from build123d import *

# Parameters (mm, degrees)
F0_W     = 203.2
F0_H     = 101.6
F1_DEPTH = 101.6
F2_W     = 101.6
F2_H     = 76.2
F3_DEPTH = 50.8
F5_DEPTH = 50.8
F7_DEPTH = 50.8


with BuildPart() as f1:
    # F0 (on Front) → F1 (new body)
    with BuildSketch(Plane.XZ):
        with Locations((-39.505829, 21.651511)):
            Rectangle(F0_W, F0_H)
    extrude(amount=F1_DEPTH)

    # F2 (on face) → F3 (cut)
    with BuildSketch(Plane.XZ.offset(101.6)):
        with Locations((-39.505829, 34.351511)):
            Rectangle(F2_W, F2_H)
    extrude(amount=-F3_DEPTH, mode=Mode.SUBTRACT)

    # F4 (on face) → F5 (cut)
    with BuildSketch(Plane.YZ.offset(-90.305829)):
        Polygon((-101.6, 72.451511), (-101.6, -3.748489), (-50.8, 72.451511), align=None)
    extrude(amount=-F5_DEPTH, mode=Mode.SUBTRACT)

    # F6 (on face) → F7 (cut)
    with BuildSketch(Plane(origin=(11.294171, 0, 0), x_dir=(0, -1, 0), z_dir=(-1, 0, 0))):
        Polygon((101.6, 72.451511), (50.8, 72.451511), (101.6, -3.748489), align=None)
    extrude(amount=-F7_DEPTH, mode=Mode.SUBTRACT)


solid = f1.part
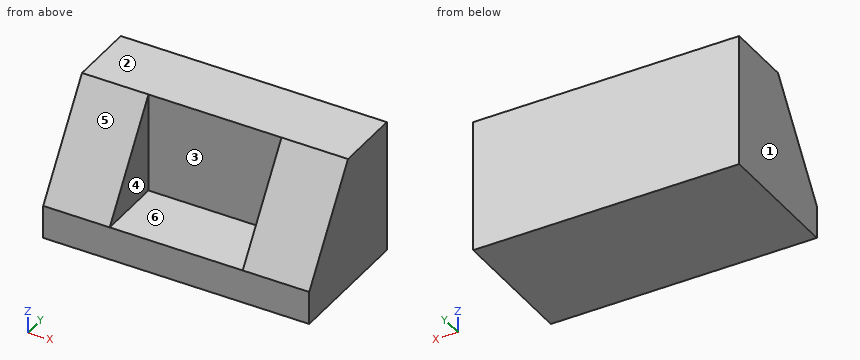
Input: part model. Units: mm. Frame: model coordinates. Face numbers are marked on the shaded views. A direction names the side the tool comes from. Give positions to 0.01 mm unless a question says otherwise; leave off trailing zeros. Loops run counter-clockwise (first coordinate to the right, second up) from the corner with the lowest first, then second, coordinate; pieces in that order, holes last. Notation, with made-up numbers: M 78.25,-2.5 L 114.25,-2.5 A29 cw 114.25,36.5 Z; hole C 45,62.5 d4. An arc over 180 degrees is marked long. Use one line per item in the form item = value.
1. Section query D-D, the plane x = -65. Return the cut outline in (y, z), and give its area (3 significant figures).
Numbers:
outline = M -101.6,-29.15 L 0,-29.15 L 0,72.45 L -50.8,72.45 L -50.8,-3.75 L -101.6,-3.75 Z
area = 6,450 mm²
2. Line query: L1, parallel to X at y = -59, z = 11; L2, parallel to Y at x = -23, z = -3; L3, parallel to Z at x = -5, y = -56. Output: solid intervals per line, ascending.
Numbers:
L1 = -141.11 to -90.31, 11.29 to 62.09
L2 = -50.8 to 0
L3 = -29.15 to -3.75
3. Section query A-A, the plane x = -100.5. Return the cut outline in (y, z), and give its area (3 significant figures).
Numbers:
outline = M -101.6,-29.15 L 0,-29.15 L 0,72.45 L -50.8,72.45 L -101.6,-3.75 Z
area = 8,390 mm²
4. Section query B-B, the plane z = 58.5. Return the cut outline in (x, y).
Numbers:
outline = M -141.11,-60.1 L -90.31,-60.1 L -90.31,-50.8 L 11.29,-50.8 L 11.29,-60.1 L 62.09,-60.1 L 62.09,0 L -141.11,0 Z
5. Section query C-C, the plane y = -65.5. Return the cut outline in (x, z).
Numbers:
outline = M -141.11,-29.15 L 62.09,-29.15 L 62.09,50.4 L 11.29,50.4 L 11.29,-3.75 L -90.31,-3.75 L -90.31,50.4 L -141.11,50.4 Z
6. Pull-direction query (X, two-part tool) for the marked faces 1, 2, 3 and 4; classes: released by +X, released by -X, zero draft, split by the parting line, or undercut.
Numbers:
face_1 = released by -X
face_2 = zero draft
face_3 = undercut
face_4 = undercut
7. Reachability of the marked faces 5 and 6 from +Z, -Z, +X, -X, +Y, -Y: full face, straight path, thin tool, end or side. Return the list, or none.
Numbers:
face_5 = +Z, +X, -X, -Y
face_6 = +Z, -Y
8. First-contact query: pin 1 (5 mm diameter, centred on x = -18.5, z = 25, fed in from -Y). Flat tip, straight axial feed; report the tip coordinate or a pass-through.
Numbers:
pin_1 = -50.8
